Geometry check sheet. Reference: the model listing, model coordinates, mm. Face numbers are marked on the shaded views. A direction names the side the tool comes from. Round coordinates to 2 decimals unless told otherwise and drop trailing zeros. Write each loop counter-clockwise with the first axis right and the second up, starting at its lowest first coordinate (ties: lowest second). Pieces come first, ordered by that corner, then holes. Notation, with made-up numbers: (56, 39.5) -> (109, 39.5) arc R15 ccw to (109, 67.5) -> close; hole circle Ø2 at (84.5, 34.25). An arc over 180 degrees is marked (long way). One line per question, with ' | ' between items.
```python
from build123d import *

# Parameters (mm, degrees)
CROQUIS1_W              = 121
CROQUIS1_H              = 10
SALIENTE_EXTRUIR1_DEPTH = 13.5
CROQUIS2_R              = 2.525
CORTAR_EXTRUIR1_DEPTH   = 8.05
CORTAR_EXTRUIR2_DEPTH   = 20
CROQUIS4_R              = 2
CORTAR_EXTRUIR3_DEPTH   = 20


with BuildPart() as part:
    # Croquis1 → Saliente-Extruir1 (new body)
    with BuildSketch(Plane(origin=(0, 0, 0), x_dir=(1, 0, 0), z_dir=(0, 1, 0))):
        with Locations((60.5, 5)):
            Rectangle(CROQUIS1_W, CROQUIS1_H)
    extrude(amount=SALIENTE_EXTRUIR1_DEPTH)

    # Croquis2 → Cortar-Extruir1 (cut)
    with BuildSketch(Plane(origin=(0, 13.5, 0), x_dir=(1, 0, 0), z_dir=(0, 1, 0))):
        with Locations((9, 5)):
            Circle(CROQUIS2_R)
        with Locations((112, 5)):
            Circle(CROQUIS2_R)
    extrude(amount=-CORTAR_EXTRUIR1_DEPTH, mode=Mode.SUBTRACT)

    # Croquis3 → Cortar-Extruir2 (cut)
    with BuildSketch(Plane.XY):
        Polygon((103, 13.5), (18, 13.5), (35.5, 8.5), (85.5, 8.5), align=None)
    extrude(amount=-CORTAR_EXTRUIR2_DEPTH, mode=Mode.SUBTRACT)

    # Croquis4 → Cortar-Extruir3 (cut)
    with BuildSketch(Plane.XY):
        with Locations((27.745, 5.76)):
            Circle(CROQUIS4_R)
        with Locations((93.255, 5.76)):
            Circle(CROQUIS4_R)
    extrude(amount=-CORTAR_EXTRUIR3_DEPTH, mode=Mode.SUBTRACT)


solid = part.part
```
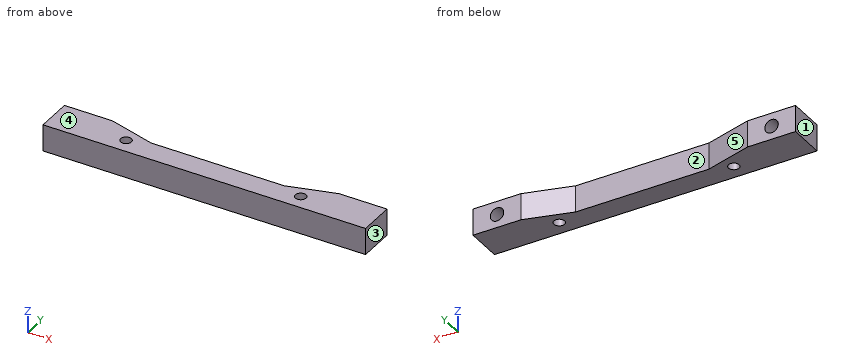
(1) Sectioned sample at D-D on x = 101.5. Record the cut outline in (y, z).
Resolved:
outline: (0, -10) -> (13.07, -10) -> (13.07, 0) -> (0, 0) -> close
(2) Sectioned sample at B-B on x = 9. Record the cut outline in (y, z) (3 decimals), then the cut area to 3 significant figures.
Resolved:
outline: (0, -10) -> (13.5, -10) -> (13.5, -7.525) -> (5.45, -7.525) -> (5.45, -2.475) -> (13.5, -2.475) -> (13.5, 0) -> (0, 0) -> close | area: 94.3 mm2
(3) Sectioned sample at C-C on x = 59.5. Record the cut outline in (y, z).
Resolved:
outline: (0, -10) -> (8.5, -10) -> (8.5, 0) -> (0, 0) -> close
(4) Draft check along X on the marked faces 3, 4 and 5. Enter one of: +X half, -X half, draft (parallel to the pull), parting line (faces both ways), or undercut.
Resolved:
face 3: +X half | face 4: draft | face 5: undercut
(5) Material ranges on line 1 (X direction, y = 5, z = -0.75); line 2 (Z direction, x = 9, y = 8) (3 decimals); line 3 (X direction, y = 4, z = -6.75), recorded low to high.
Resolved:
line 1: x = 0 to 25.9, 29.59 to 91.41, 95.1 to 121 | line 2: z = -10 to -7.525, -2.475 to 0 | line 3: x = 0 to 26.8, 28.69 to 92.31, 94.2 to 121
(6) Sectioned sample at A-A on z = -5. Record the cut outline in (x, y) (3 decimals).
Resolved:
outline: (0, 0) -> (121, 0) -> (121, 13.5) -> (114.525, 13.5) -> (114.525, 5.45) -> (109.475, 5.45) -> (109.475, 13.5) -> (103, 13.5) -> (85.5, 8.5) -> (35.5, 8.5) -> (18, 13.5) -> (11.525, 13.5) -> (11.525, 5.45) -> (6.475, 5.45) -> (6.475, 13.5) -> (0, 13.5) -> close; hole circle Ø4 at (27.745, 5.76); hole circle Ø4 at (93.255, 5.76)
(7) Access from +Z, -Z, +X, -X, +Y, -Y to the whole of each face (thin tool, end or side, straight path). Record for the marked faces 1 and 2.
Resolved:
face 1: +Z, -Z, -X, +Y, -Y | face 2: +Z, -Z, +Y
(8) Go/stop test with flat-tipped pins: pin 1 (2 mm diameter, centred on x = 22.5, z = -8, fed in from +Y); pin 2 (1.5 mm diameter, centred on x = 9.5, z = -6, fed in from +Y). Record where each tip stops, or that it passes through.
Resolved:
pin 1: stops at y = 12.5 | pin 2: stops at y = 5.45
